Read the model definition and answer for the solid it produces. Units are mm, in the model's axes. Coordinates: 2 decimals unless noted, no trailing zeros. Order: outer loops, then holes, each group sorted by start corner. A loop starts at its lowest first (then second) coordinate and runs counter-clockwise, first axis right, second up. Notation, with made-up numbers: (74.25, 25.5) - (123.25, 25.5) arc R24 cw to (123.25, 47.5) - close; hole circle Ø4 at (32.25, 50.5). An arc over 180 degrees is marked (long way). Answer as a JSON object with one key per item and string values. Group by question number.
from build123d import *

# Parameters (mm, degrees)
SKETCH1_R           = 2
BOSS_EXTRUDE1_DEPTH = 7.5
CUT_EXTRUDE1_DEPTH  = 2
CHAMFER1_SIZE       = 0.2


with BuildPart() as part:
    # Sketch1 → Boss-Extrude1 (new, symmetric)
    with BuildSketch(Plane(origin=(0, 0, 0), x_dir=(1, 0, 0), z_dir=(0, 1, 0))):
        with Locations(Location((0, 0, 0), (0, 0, 270))):
            Circle(SKETCH1_R)
    extrude(amount=BOSS_EXTRUDE1_DEPTH, both=True)

    # Sketch2 → Cut-Extrude1 (cut)
    with BuildSketch(Plane(origin=(0, 7.5, 0), x_dir=(1, 0, 0), z_dir=(0, 1, 0))):
        Polygon((0.721687836, 1.25), (-0.721687836, 1.25), (-1.443375673, 0), (-0.721687836, -1.25), (0.721687836, -1.25), (1.443375673, 0), align=None)
    extrude(amount=-CUT_EXTRUDE1_DEPTH, mode=Mode.SUBTRACT)

    # Chamfer1
    chamfer1_edges = [part.edges().sort_by_distance(p)[0] for p in [
        (0, 7.5, -2),
    ]]
    chamfer(chamfer1_edges, length=CHAMFER1_SIZE)


solid = part.part
1. A cutting plane is placed at A-A on y = 6.75. Write down the section's boundary in (x, z), and give its area (3 significant figures).
2. A cutting plane is placed at C-C on y = 1.75. Write down the section's boundary in (x, z).
3. Given pin 1 (1.5 mm diameter, centred on y = -4, z = -1, fed in from -X); pin 2 (1 mm diameter, centred on x = 0.5, z = -0.5, fed in from +Y), each flat-ended and moving along its own axis, determine where each tip first touches the part or whether it passes through.
4. Straight lines are drawn through the part: L1, parallel to X at y = 6.5, z = 1.15; L2, parallel to Z at x = -1.35, y = 6.5; L3, parallel to Y at x = -0.05, z = 0.75. For each, find the intervals that lie inside material, in ascending order.
5. For a pull along X with two mould halves and no side action, classify faces 1 (the flat face through (-1.08, 6.51, -0.63)), 2 (the flat face through (-1.088, 6.514, 0.616)), 3 (the cylindrical face through (-2, 0, 0)), 4 (the flat face through (0, -7.5, 0)) as pulls with the +X half, pulls with the -X half, needs draft (parallel to the pull), parting line crosses it, or undercut.
6. A cutting plane is placed at B-B on x = 0. Write down the section's boundary in (y, z), and give its area (3 significant figures).
Derived:
{
 "1": {"outline": "circle Ø4 at (0, 0); hole (-1.44, 0) - (-0.72, -1.25) - (0.72, -1.25) - (1.44, 0) - (0.72, 1.25) - (-0.72, 1.25) - close", "area": "7.15 mm2"},
 "2": {"outline": "circle Ø4 at (0, 0)"},
 "3": {"pin 1": "stops at x = -1.98", "pin 2": "stops at y = 5.5"},
 "4": {"L1": "x = -1.64 to -0.78, 0.78 to 1.64", "L2": "z = -1.48 to -0.16, 0.16 to 1.48", "L3": "y = -7.5 to 5.5"},
 "5": {"face 1": "undercut", "face 2": "undercut", "face 3": "parting line crosses it", "face 4": "needs draft"},
 "6": {"outline": "(-7.5, -2) - (7.3, -2) - (7.5, -1.8) - (7.5, -1.25) - (5.5, -1.25) - (5.5, 1.25) - (7.5, 1.25) - (7.5, 1.8) - (7.3, 2) - (-7.5, 2) - close", "area": "55.0 mm2"}
}
